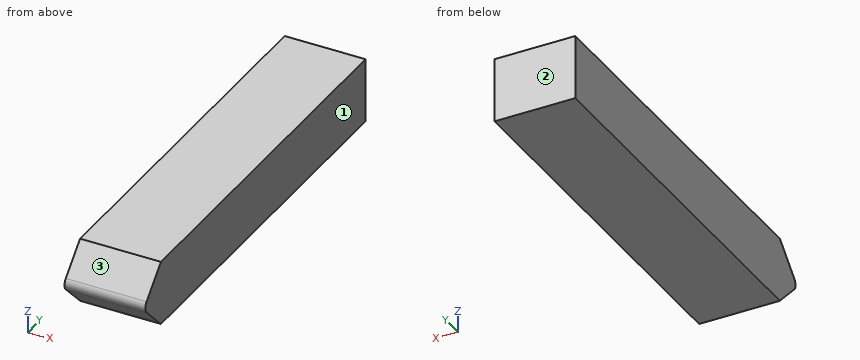
from build123d import *

# Parameters (mm, degrees)
BOSS_EXTRUDE1_DEPTH = 25.4
FILLET1_R           = 2.54


with BuildPart() as part:
    # Sketch1 → Boss-Extrude1 (new body)
    with BuildSketch(Plane(origin=(0, 0, 0), x_dir=(0, 0, -1), z_dir=(1, 0, 0))):
        Polygon((-10.16, 0), (-10.16, -119.38), (0, -129.54), (10.16, -119.38), (10.16, 0), align=None)
    extrude(amount=BOSS_EXTRUDE1_DEPTH)

    # Fillet1
    fillet1_edges = [part.edges().sort_by_distance(p)[0] for p in [
        (12.7, -129.54, 0),
    ]]
    fillet(fillet1_edges, radius=FILLET1_R)


solid = part.part
Model file for the job. Use its own axes, mm. Face numbers are marked on the shaded views. Give positions to 0.01 mm unless a question says otherwise; leave off trailing zeros. Order: outer loops, then holes, each group sorted by start corner. A loop starts at its lowest first (then second) coordinate and runs counter-clockwise, first axis right, second up. Notation, with made-up numbers: (-35.5, 78.5) -> (17.5, 78.5) arc R18 cw to (17.5, 99.5) -> close; hole circle Ø4 at (82, 82.5). An arc over 180 degrees is marked (long way). Use CSV: the item, a comma, the result in double quotes.
1. Band-saw the part on C-C, the plane z = 4. Give the cut face in (x, y).
Outcome:
outline,"(0, -125.54) -> (25.4, -125.54) -> (25.4, 0) -> (0, 0) -> close"
2. Drop a flat-ended pin along its axis: pin 1 (5 mm diameter, centred on x = 18, z = -3.5, fed in from -Y). Give the stop position or say it passes through.
Outcome:
pin 1,"y = -128.28"
3. Band-saw the part on A-A, the plane x = 13.5. Give the cut face in (y, z), then the cut area to 3 significant figures.
Outcome:
outline,"(-127.74, -1.8) -> (-119.38, -10.16) -> (0, -10.16) -> (0, 10.16) -> (-119.38, 10.16) -> (-127.74, 1.8) arc R2.54 ccw to start"
area,"2,530 mm²"
4. Drill centre lines: line 1 along Y through (x, z) = (10.25, -5.5); line 2 along Y through (x, z) = (17.25, 7). Where is each one in solid material? Low to high. Write a range as from..to.
Outcome:
line 1,"-124.04..0"
line 2,"-122.54..0"
5. Band-saw the part on B-B, the plane z = -3.25. Give the cut face in (x, y).
Outcome:
outline,"(0, -126.29) -> (25.4, -126.29) -> (25.4, 0) -> (0, 0) -> close"
6. Mould opens along Y. For the marked faces 1, 2 and 3 say: +Y half, -Y half, draft (parallel to the pull), parting line (faces both ways), or undercut.
Outcome:
face 1,"draft"
face 2,"+Y half"
face 3,"-Y half"
